Could you check a few things on this drawing? It's one solid part, dimensions in mm from its lowest x, y, z. Round coordinates to 2 decimals unless told otherwise and drop trailing zeros. Loops run counter-clockwise (first coordinate to the right, second up) from the corner with the lowest first, then second, coordinate; pieces in that order, holes last. Notation, with made-up numbers: M 36,82.25 L 60,82.25 A34 ccw 60,119.25 Z; hole C 86,-4 d2. An arc over 180 degrees is marked long. Return JSON: item names as keys, results as strings.
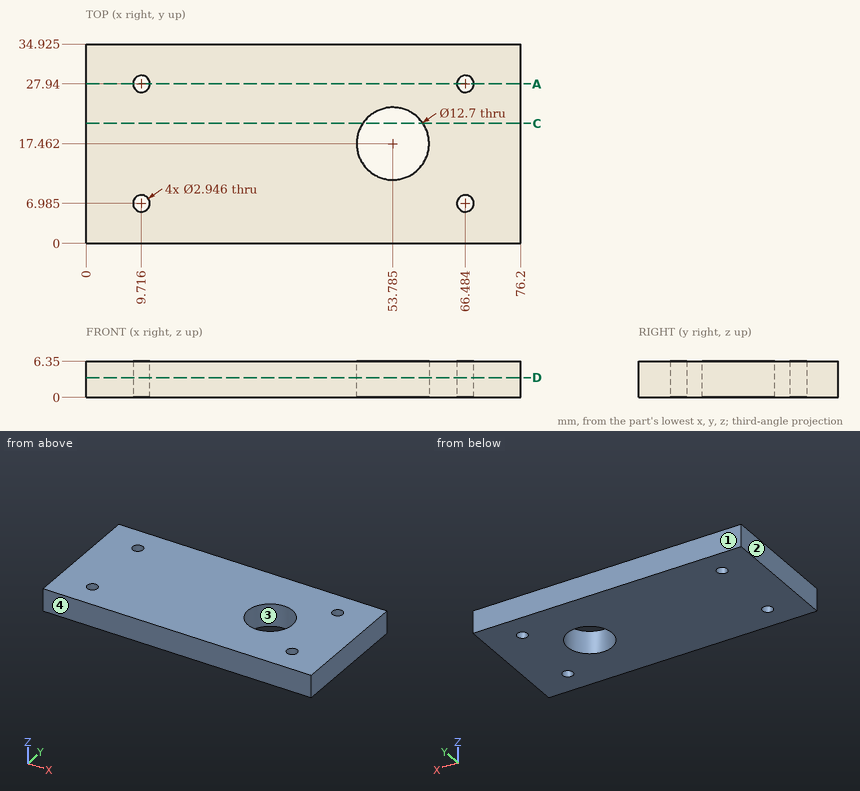
Q1. Suppose I cut it at A-A, the plane y = 27.94. Please give me the cut outline in (x, z).
Results:
{"outline": "M 0,0 L 8.24,0 L 8.24,6.35 L 0,6.35 Z; M 11.19,0 L 65.01,0 L 65.01,6.35 L 11.19,6.35 Z; M 67.96,0 L 76.2,0 L 76.2,6.35 L 67.96,6.35 Z"}
Q2. Suppose I cut it at D-D, the plane z = 3.5. State how many separate pieces and enclosed holes the cut face has, plus the area to 3 significant figures.
Results:
{"separate pieces": "1", "enclosed holes": "5", "area": "2,510 mm2"}
Q3. If I drill on line 1 along Y through (x, z) = (9.5, 6) (1 decimal); line 2 along X through (y, z) = (17, 4); line 3 along X through (y, z) = (17.5, 1.5) (1 decimal), over which ranges is the centre line in solid material (lowest first)?
Results:
{"line 1": "y = 0 to 5.5, 8.4 to 26.5, 29.4 to 34.9", "line 2": "x = 0 to 47.45, 60.12 to 76.2", "line 3": "x = 0 to 47.4, 60.1 to 76.2"}
Q4. I'm going to push a flat-ended pin straight in: pin 1 Ø1.5 at (x, y) = (9.5, 28.5) entering from -Z. Where does the tip first touch, or does it pass through?
Results:
{"pin 1": "passes through"}
Q5. Suppose I cut it at C-C, the plane y = 21. Please give me the cut outline in (x, z).
Results:
{"outline": "M 0,0 L 48.51,0 L 48.51,6.35 L 0,6.35 Z; M 59.06,0 L 76.2,0 L 76.2,6.35 L 59.06,6.35 Z"}
Q6. Thinking about a two-plate mould opening in Y: for the marked faces 1, 2, 3 and 4, which applies, pulls with the +Y half, pulls with the -Y half, needs draft (parallel to the pull), parting line crosses it, or undercut?
Results:
{"face 1": "pulls with the +Y half", "face 2": "needs draft", "face 3": "undercut", "face 4": "pulls with the -Y half"}
